```python
from build123d import *


with BuildPart() as f1:
    # F0 (on Front) → F1 (revolve)
    with BuildSketch(Plane.XZ):
        with BuildLine():
            Line((-25.4, 0), (0, 0))
            Line((0, 0), (0, 6.35))
            ThreePointArc((0, 6.35), (-2.795959, 8.87707), (0, 11.404141))
            Line((0, 11.404141), (0, 39.390257))
            ThreePointArc((0, 39.390257), (-2.313396, 41.920128), (0, 44.45))
            Line((0, 44.45), (0, 50.8))
            Line((0, 50.8), (-25.4, 50.8))
            Line((-25.4, 50.8), (-25.4, 0))
        make_face()
    revolve(axis=Axis((-25.4, 0, 25.4), (0, 0, 1)))


solid = f1.part
```
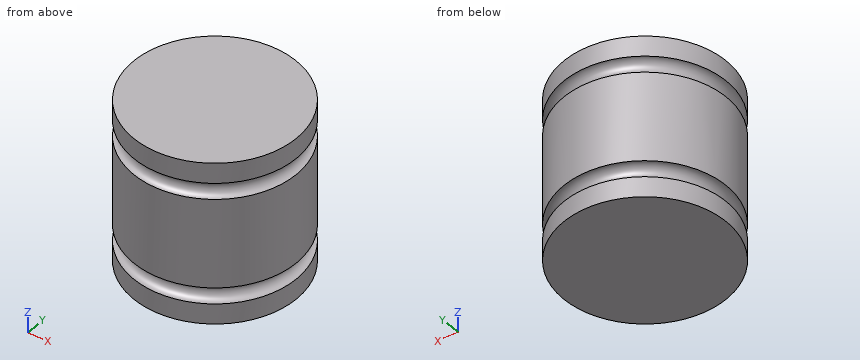
The model under review builds one solid part; all positions refer to its coordinate system, in mm. Round coordinates to 2 decimals unless told otherwise and drop trailing zeros. Order: outer loops, then holes, each group sorted by start corner. A loop starts at its lowest first (then second) coordinate and runs counter-clockwise, first axis right, second up. Notation, with made-up numbers: (-2.5, 63.25) - (23.5, 63.25) arc R18 cw to (23.5, 91.25) - close; hole circle Ø6 at (58, 60). An arc over 180 degrees is marked (long way). Answer in a Markdown table with one row per item.
(1) Take a section at C-C on z = 46.5. Write out the cut boundary in (x, y), plus the area to 3 significant figures.
Result set:
| item | result |
|---|---|
| outline | circle Ø50.8 at (-25.4, 0) |
| area | 2,030 mm2 |
(2) Take a section at A-A on y = 0. Write out the cut boundary in (x, z), plus the area to 3 significant figures.
Result set:
| item | result |
|---|---|
| outline | (-50.8, 0) - (0, 0) - (0, 6.35) arc R2.54 cw (long way) to (0, 11.4) - (0, 39.39) arc R2.54 cw to (0, 44.45) - (0, 50.8) - (-50.8, 50.8) - (-50.8, 44.45) arc R2.54 cw to (-50.8, 39.39) - (-50.8, 11.4) arc R2.54 cw (long way) to (-50.8, 6.35) - close |
| area | 2,540 mm2 |
(3) Take a section at B-B on x = -25.4. Write out the cut boundary in (y, z).
Result set:
| item | result |
|---|---|
| outline | (-25.4, 0) - (25.4, 0) - (25.4, 6.35) arc R2.54 cw (long way) to (25.4, 11.4) - (25.4, 39.39) arc R2.54 cw to (25.4, 44.45) - (25.4, 50.8) - (-25.4, 50.8) - (-25.4, 44.45) arc R2.54 cw to (-25.4, 39.39) - (-25.4, 11.4) arc R2.54 cw (long way) to (-25.4, 6.35) - close |
(4) For line 1 (Z direction, x = -15, y = -21); line 2 (Z direction, x = -39, y = 20); line 3 (Y direction, x = -25, z = 26), list the stretches that pass through material, from the lowest coordinate up. Write a range as from..to.
Result set:
| item | result |
|---|---|
| line 1 | z = 0..7, 10.76..40.64, 43.2..50.8 |
| line 2 | z = 0..6.52, 11.23..39.83, 44.01..50.8 |
| line 3 | y = -25.4..25.4 |
(5) Clearance check with flat-ended pins moving along their axes: P1, Ø10, axis at x = -45.5, z = 43.5, coming from the +Y side; P2, Ø10, axis at y = 16.5, z = 31.5, coming from the -X side; P3, Ø4, axis at x = -42, z = 12.5, coming from the -Y side. State where each tip first meets the part, or that it passes through.
Result set:
| item | result |
|---|---|
| P1 | stops at y = 20.36 |
| P2 | stops at x = -48.05 |
| P3 | stops at y = -20.78 |
